Geometry check sheet. Reference: drawing and pictorial views, mm from the part's lowest x, y, z. Coordinates: 2 decimals unless noted, no trailing zeros. Loops run counter-clockwise (first coordinate to the right, second up) from the corner with the lowest first, then second, coordinate; pieces in that order, holes last. Notation, with made-up numbers: (-11, 25.25) - (29, 25.25) arc R26 cw to (29, 43.25) - close; hole circle Ø11 at (72.25, -20.75). An arc over 180 degrees is marked (long way). One line per item, written item: value.
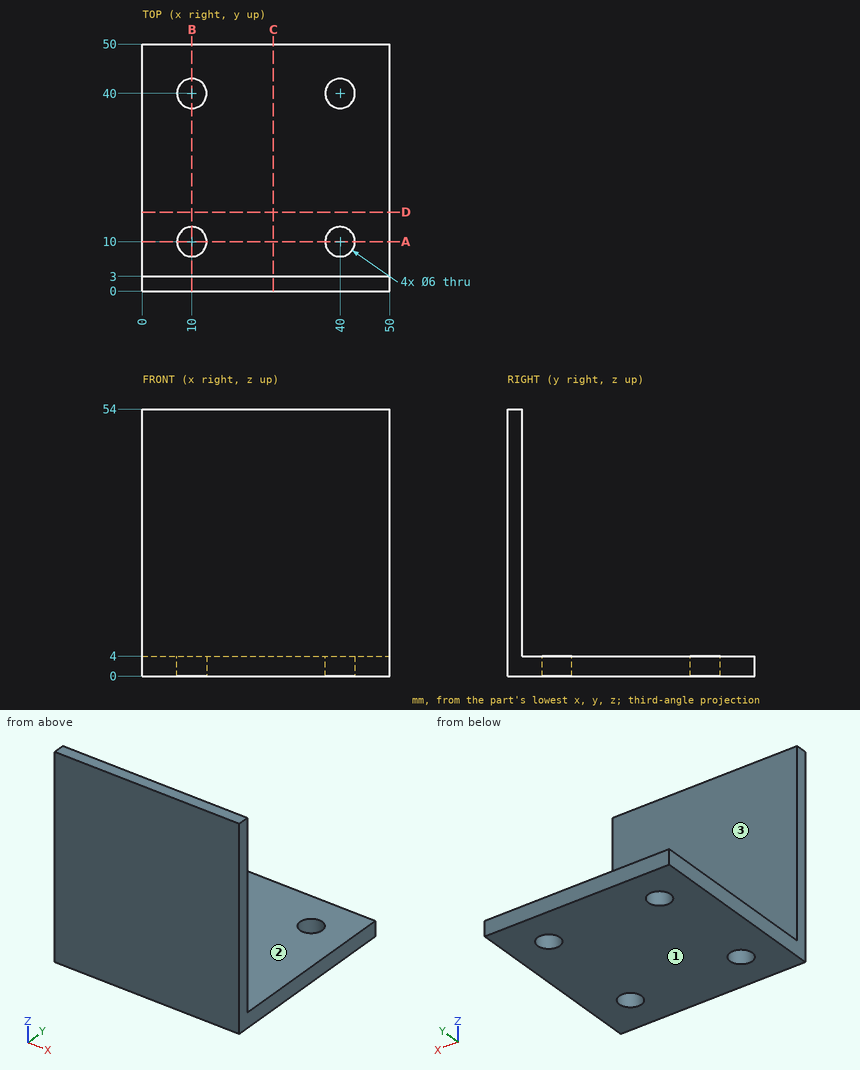
(1) Cross-section at C-C on x = 26.5. Record the cut outline in (y, z).
Reply:
outline: (0, 0) - (50, 0) - (50, 4) - (3, 4) - (3, 54) - (0, 54) - close
(2) Cross-section at D-D on y = 16. Record the cut outline in (x, z).
Reply:
outline: (0, 0) - (50, 0) - (50, 4) - (0, 4) - close
(3) Cross-section at B-B on x = 10. Record the cut outline in (y, z).
Reply:
outline: (0, 0) - (7, 0) - (7, 4) - (3, 4) - (3, 54) - (0, 54) - close; (13, 0) - (37, 0) - (37, 4) - (13, 4) - close; (43, 0) - (50, 0) - (50, 4) - (43, 4) - close
(4) Release check for a two-part mould opening along Z. For the marked faces 1, 2 and 3 record: pulls with the +Z half, pulls with the -Z half, needs draft (parallel to the pull), parting line crosses it, or undercut.
Reply:
face 1: pulls with the -Z half
face 2: pulls with the +Z half
face 3: needs draft
(5) Cross-section at A-A on y = 10. Record the cut outline in (x, z), and give its area (3 significant figures).
Reply:
outline: (0, 0) - (7, 0) - (7, 4) - (0, 4) - close; (13, 0) - (37, 0) - (37, 4) - (13, 4) - close; (43, 0) - (50, 0) - (50, 4) - (43, 4) - close
area: 152 mm2
(6) Material ranges on probe 1 along Y at (x, z) = (40, 2); probe 2 along Z at (x, y) = (44, 31.5); probe 3 along Y at (x, z) = (3.5, 4.5), recorded low to high. Write a range as from..to.
Reply:
probe 1: 0..7, 13..37, 43..50
probe 2: 0..4
probe 3: 0..3
(7) Go/stop test with flat-tipped pins: pin 1 Ø15 at (x, z) = (31, 20) entering from +Y; pin 2 Ø5 at (x, y) = (39.5, 14.5) entering from +Z. Record where each tip stops, or that it passes through.
Reply:
pin 1: y = 3
pin 2: z = 4
